Can you work these out from the model? Positions are in its coordinate system, mm. A direction names the side the tool comes from. Round coordinates to 2 decimals unless told otherwise and drop trailing zeros. Loops run counter-clockwise (first coordinate to the right, second up) from the corner with the lowest first, then second, coordinate; pieces in that order, holes last. Notation, with made-up numbers: (4.5, 41) -> (62.5, 41) arc R20 ccw to (62.5, 64) -> close; hole circle Ø5 at (-2.75, -15). An arc over 180 degrees is marked (long way). Answer as a JSON object with one key per item and string values.
```python
from build123d import *

# Parameters (mm, degrees)
EXTRUDE_THIN1_DEPTH  = 30
CONVERT_SOLID1_START = -20
CONVERT_SOLID1_DEPTH = 20


# Read off the part's stored shape, not the designer's step: Convert-Solid1
with BuildPart() as part:
    # Sketch1 → Extrude-Thin1 (new body)
    with BuildSketch(Plane(origin=(0, 0, 0), x_dir=(1, 0, 0), z_dir=(0, 1, 0))):
        with BuildLine():
            Line((0.5, 63.5), (32.11260948, 63.5))
            ThreePointArc((32.11260948, 63.5), (40.836461979, 59.886461979), (44.45, 51.16260948))
            Line((44.45, 51.16260948), (44.45, -38.1))
            ThreePointArc((44.45, -38.1), (37.010512242, -56.060512242), (19.05, -63.5))
            Line((19.05, -63.5), (-19.05, -63.5))
            ThreePointArc((-19.05, -63.5), (-37.010512242, -56.060512242), (-44.45, -38.1))
            Line((-44.45, -38.1), (-44.45, 51.16260948))
            ThreePointArc((-44.45, 51.16260948), (-40.836461979, 59.886461979), (-32.11260948, 63.5))
            Line((-32.11260948, 63.5), (-0.5, 63.5))
            Line((-0.5, 63.5), (-0.5, 61.9125))
            Line((-0.5, 61.9125), (-32.11260948, 61.9125))
            ThreePointArc((-32.11260948, 61.9125), (-39.713929964, 58.763929964), (-42.8625, 51.16260948))
            Line((-42.8625, 51.16260948), (-42.8625, -38.1))
            ThreePointArc((-42.8625, -38.1), (-35.887980227, -54.937980227), (-19.05, -61.9125))
            Line((-19.05, -61.9125), (19.05, -61.9125))
            ThreePointArc((19.05, -61.9125), (35.887980227, -54.937980227), (42.8625, -38.1))
            Line((42.8625, -38.1), (42.8625, 51.16260948))
            ThreePointArc((42.8625, 51.16260948), (39.713929964, 58.763929964), (32.11260948, 61.9125))
            Line((32.11260948, 61.9125), (0.5, 61.9125))
            Line((0.5, 61.9125), (0.5, 63.5))
        make_face()
    extrude(amount=EXTRUDE_THIN1_DEPTH)

    # Convert-Solid1 outline → Convert-Solid1 (add)
    with BuildSketch(Plane(origin=(0, 0, 0), x_dir=(1, 0, 0), z_dir=(0, 1, 0)).offset(CONVERT_SOLID1_START)):
        with BuildLine():
            Line((0.5, 61.9125), (32.11260948, 61.9125))
            ThreePointArc((32.11260948, 61.9125), (39.713929964, 58.763929964), (42.8625, 51.16260948))
            Line((42.8625, 51.16260948), (42.8625, -38.1))
            ThreePointArc((42.8625, -38.1), (35.887980227, -54.937980227), (19.05, -61.9125))
            Line((19.05, -61.9125), (-19.05, -61.9125))
            ThreePointArc((-19.05, -61.9125), (-35.887980227, -54.937980227), (-42.8625, -38.1))
            Line((-42.8625, -38.1), (-42.8625, 51.16260948))
            ThreePointArc((-42.8625, 51.16260948), (-39.713929964, 58.763929964), (-32.11260948, 61.9125))
            Line((-32.11260948, 61.9125), (-0.5, 61.9125))
            Line((-0.5, 61.9125), (-0.5, 63.5))
            Line((-0.5, 63.5), (-32.11260948, 63.5))
            ThreePointArc((-32.11260948, 63.5), (-40.836461979, 59.886461979), (-44.45, 51.16260948))
            Line((-44.45, 51.16260948), (-44.45, -38.1))
            ThreePointArc((-44.45, -38.1), (-37.010512242, -56.060512242), (-19.05, -63.5))
            Line((-19.05, -63.5), (19.05, -63.5))
            ThreePointArc((19.05, -63.5), (37.010512242, -56.060512242), (44.45, -38.1))
            Line((44.45, -38.1), (44.45, 51.16260948))
            ThreePointArc((44.45, 51.16260948), (40.836461979, 59.886461979), (32.11260948, 63.5))
            Line((32.11260948, 63.5), (0.5, 63.5))
            Line((0.5, 63.5), (0.5, 61.9125))
        make_face()
    extrude(amount=CONVERT_SOLID1_DEPTH)


solid = part.part
```
Q1. I'm going to push flat-ended pins straight in: pin 1 (12 mm diameter, centred on y = 2, z = 50.5, fed in from +X); pin 2 (0.8 mm diameter, centred on y = 17, z = -63, fed in from -X); pin 3 (0.5 mm diameter, centred on y = 5.5, z = -62.5, fed in from +X). Where does each tip first touch, or does it pass through?
Determined:
{"pin 1": "x = 43.63", "pin 2": "x = -36.74", "pin 3": "x = 37.52"}
Q2. I want a section at A-A, the plane x = -14. Write out the boundary of the cut face in (y, z), then the cut area to 3 significant figures.
Determined:
{"outline": "(-20, -63.5) -> (30, -63.5) -> (30, -61.91) -> (-20, -61.91) -> close; (-20, 61.91) -> (30, 61.91) -> (30, 63.5) -> (-20, 63.5) -> close", "area": "159 mm²"}
Q3. We'd pull the mould along Z, two halves only. Please class faces 3 (the flat face through (-17, 5, -61.912)), 4 (the flat face through (-16, 5, -63.5)), 5 (the flat face through (0, 5, 63.5)), 6 (the flat face through (44.45, 5, -6)): pulls with the +Z half, pulls with the -Z half, needs draft (parallel to the pull), parting line crosses it, or undercut.
Determined:
{"face 3": "undercut", "face 4": "pulls with the -Z half", "face 5": "pulls with the +Z half", "face 6": "needs draft"}
Q4. If I drill on L1, parallel to X at y = -18, z = -48; L2, parallel to Z at x = 6, y = 4.5; L3, parallel to X at y = 7.5, z = 44.5, over which ranges is the centre line in solid material (lowest first)? Write a range as [from, to].
Determined:
{"L1": "[-44.45, -42.86], [42.86, 44.45]", "L2": "[-63.5, -61.91], [61.91, 63.5]", "L3": "[-43.63, -41.99], [41.99, 43.63]"}
Q5. On a 3-axis mill with a long thin cutter (end or side, diameter ignored), from which of +Z, -Z, +X, -X, +Y, -Y can I reach the whole of each face in a straight line? I mean faces 1 (the flat face through (16, 5, -61.912)), 2 (the cylindrical face through (40.93, 4.65, -59.79)). Say none if no direction works.
Determined:
{"face 1": "+Y, -Y", "face 2": "-Z, +X, +Y, -Y"}
Q6. I want a section at B-B, the plane z = 4.5. Write out the boundary of the cut face in (x, y), then the cut area to 3 significant figures.
Determined:
{"outline": "(-44.45, -20) -> (-42.86, -20) -> (-42.86, 30) -> (-44.45, 30) -> close; (42.86, -20) -> (44.45, -20) -> (44.45, 30) -> (42.86, 30) -> close", "area": "159 mm²"}
